CAD build for the part. Positions are in the model's coordinates, mm. Face numbers are marked on the shaded views. Give positions to 0.01 mm unless a question says otherwise; leave off trailing zeros. Loops run counter-clockwise (first coordinate to the right, second up) from the corner with the lowest first, then second, coordinate; pieces in that order, holes last.
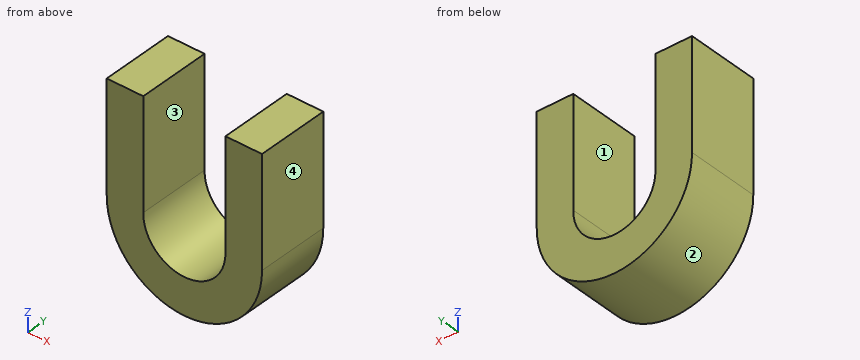
```python
from build123d import *

# Parameters (mm, degrees)
F1_DEPTH = 25.4


with BuildPart() as f1:
    # F0 (on Front) → F1 (new body)
    with BuildSketch(Plane.XZ):
        with BuildLine():
            ThreePointArc((14.285613, 0.232226), (0, -14.2875), (-14.285613, 0.232226))
            Line((-14.285613, 0.232226), (-14.285613, 38.332226))
            Line((-14.285613, 38.332226), (-26.986805, 38.332226))
            Line((-26.986805, 38.332226), (-26.986805, 0.232226))
            ThreePointArc((-26.986805, 0.232226), (0, -26.94898), (26.986805, 0.232226))
            Line((26.986805, 0.232226), (26.988195, 0.232226))
            Line((26.988195, 0.232226), (26.988195, 38.332226))
            Line((26.988195, 38.332226), (14.289387, 38.332226))
            Line((14.289387, 38.332226), (14.289387, 0.232226))
            Line((14.289387, 0.232226), (14.285613, 0.232226))
        make_face()
    extrude(amount=F1_DEPTH)


solid = f1.part
```
1. Drop flat-ended pins along their axis: pin 1 (3 mm diameter, centred on x = -16, z = 28, fed in from +Y); pin 2 (1 mm diameter, centred on y = -13.5, z = -12, fed in from -X); pin 3 (12 mm diameter, centred on x = -5, z = 12.5, fed in from -Y); pin 4 (1.5 mm diameter, centred on x = 11, y = -6, fed in from -Z). Give the stop position or say it passes through.
Responses:
pin 1: stops at y = 0
pin 2: stops at x = -24.4
pin 3: passes through
pin 4: stops at z = -24.93
2. Saw through at C-C, the plane x = 0. List the corners of the cut face in (y, z).
Responses:
outline: (-25.4, -26.95) - (0, -26.95) - (0, -14.29) - (-25.4, -14.29) - close
3. Pull direction X, two halves, no side cores. Call the marked faces 1, 2, 3 and 4: released by +X, released by -X, zero draft, split by the parting line, or undercut.
Responses:
face 1: undercut
face 2: split by the parting line
face 3: undercut
face 4: released by +X
4. Saw through at B-B, the plane z = -13.5. List the corners of the cut face in (x, y).
Responses:
outline: (-23.35, -25.4) - (-4.68, -25.4) - (-4.68, 0) - (-23.35, 0) - close; (4.68, -25.4) - (23.35, -25.4) - (23.35, 0) - (4.68, 0) - close
5. Probe line 1 along X through (y, z) = (-4.75, 18.5); line 2 along X through (y, z) = (-11, -13); line 3 along Z through (x, y) = (21, -11). List the from-to ranges inside material, lowest first.
Responses:
line 1: x = -26.99 to -14.29, 14.29 to 26.99
line 2: x = -23.63 to -5.93, 5.93 to 23.63
line 3: z = -16.91 to 38.33
6. Saw through at D-D, the plane x = 18. List the corners of the cut face in (y, z).
Responses:
outline: (-25.4, -20.07) - (0, -20.07) - (0, 38.33) - (-25.4, 38.33) - close
